Solid Edge part; units mm, degrees
sketch "Sketch1" plane through (0, 0, 0) normal (0, -1, 0) x (1, 0, 0)
  line L0 (-22.5, 45) -> (22.5, 45)
  line L1 (22.5, 45) -> (22.5, 0)
  line L2 (22.5, 0) -> (-22.5, 0)
  line L3 (-22.5, 0) -> (-22.5, 45)
  dimension "D1" = 22.5
  dimension "D2" = 22.5
  dimension "D3" = 22.5
  dimension "D4" = 22.5
extrude "Protrusion1" add sketch "Sketch1" against normal blind 270
sketch "Sketch2" plane through (22.5, 276.5897, 32.5) normal (1, 0, 0) x (0, 1, 0)
  line L0 (-86.5897, -22.5) -> (-86.5897, -32.5)
  line L1 (-86.5897, -32.5) -> (-6.5897, -32.5)
  line L2 (-6.5897, -22.5) -> (-6.5897, -32.5)
  line L3 (-86.5897, -22.5) -> (-6.5897, -22.5)
  line L4 (-276.5897, -22.5) -> (-276.5897, -32.5)
  line L5 (-196.5897, -32.5) -> (-276.5897, -32.5)
  line L6 (-196.5897, -32.5) -> (-196.5897, -22.5)
  line L7 (-196.5897, -22.5) -> (-276.5897, -22.5)
  dimension "D1" = 86.5897
  dimension "D2" = 86.5897
extrude "ExtrudedProtrusion_3" add sketch "Sketch2" along normal blind 65
sketch "Sketch3" plane through (50, 0, 15) normal (0, -1, 0) x (1, 0, 0)
  line L0 (-60, 17.5) -> (-60, 12.5)
  line L1 (-60, 12.5) -> (-55, 12.5)
  line L2 (-55, 12.5) -> (-55, 17.5)
  line L3 (-55, 17.5) -> (-60, 17.5)
extrude "ExtrudedProtrusion_5" add sketch "Sketch3" along normal blind 14.1229
sketch "Sketch4" plane through (0, -7.0615, 32.5) normal (0, 0, 1) x (0, 1, 0)
  line L0 (-7.0615, 10) -> (-7.0615, 5)
  line L1 (-7.0615, 5) -> (-2.0615, 5)
  line L2 (-2.0615, 5) -> (-2.0615, 10)
  line L3 (-2.0615, 10) -> (-7.0615, 10)
  dimension "D1" = 2.0615
extrude "ExtrudedProtrusion_6" add sketch "Sketch4" along normal blind 90
sketch "Sketch5" plane through (0, -9.1229, 61.3303) normal (0, 1, 0) x (0, 0, -1)
  line L0 (-61.1697, 10) -> (-61.1697, 5)
  line L1 (-61.1697, 5) -> (-56.1697, 5)
  line L2 (-56.1697, 5) -> (-56.1697, 10)
  line L3 (-56.1697, 10) -> (-61.1697, 10)
  dimension "D1" = 56.1697
extrude "ExtrudedProtrusion_7" add sketch "Sketch5" along normal blind 100
sketch "Sketch6" plane through (50, 270, 15) normal (0, 1, 0) x (0, 0, -1)
  line L0 (-17.5, 55) -> (-12.5, 55)
  line L1 (-12.5, 55) -> (-12.5, 60)
  line L2 (-17.5, 60) -> (-12.5, 60)
  line L3 (-17.5, 55) -> (-17.5, 60)
  dimension "D1" = 17.5
  dimension "D2" = 17.5
  dimension "D3" = 17.5
extrude "ExtrudedProtrusion_8" add sketch "Sketch6" along normal blind 14.2
sketch "Sketch7" plane through (0, 377.1, 32.5) normal (0, 0, 1) x (0, 1, 0)
  line L0 (-97.9, 10) -> (-92.9, 10)
  line L1 (-92.9, 10) -> (-92.9, 5)
  line L2 (-92.9, 5) -> (-97.9, 5)
  line L3 (-97.9, 5) -> (-97.9, 10)
  dimension "D1" = 97.9
  dimension "D2" = 92.9
extrude "ExtrudedProtrusion_9" add sketch "Sketch7" along normal blind 90
sketch "Sketch8" plane through (0, 279.2, 62.5) normal (0, -1, 0) x (0, 0, 1)
  line L0 (55, 10) -> (60, 10)
  line L1 (60, 10) -> (60, 5)
  line L2 (60, 5) -> (55, 5)
  line L3 (55, 5) -> (55, 10)
  dimension "D1" = 55
  dimension "D2" = 60
extrude "ExtrudedProtrusion_10" add sketch "Sketch8" along normal blind 100
sketch "Sketch9" plane through (-22.5, 185, 15) normal (-1, 0, 0) x (0, 1, 0)
  line L0 (-60, 15) -> (-60, -30)
  line L1 (-60, -30) -> (-40, -30)
  line L2 (-40, -30) -> (-40, 15)
  line L3 (-40, 15) -> (-60, 15)
  dimension "D1" = 60
  dimension "D2" = 40
extrude "ExtrudedProtrusion_11" add sketch "Sketch9" along normal blind 90
hole "Hole_1" at (-87.5, 125, 22.5) direction (0, 1, 0) diameter 30 end up to next
fillet "Round_1" radius 10 2 edges at (-112.5, 135, 0) (-112.5, 135, 45)
hole "Hole_2" at (-5, -11.6229, 75) direction (-1, 0, 0) diameter 3 end up to next
extrude "Protrusion2" [suppressed]
Work out the finished part from the listing and answer in its coordinate system (mm). A direction names the side the tool comes from. Round coordinates to 2 decimals unless told otherwise and drop trailing zeros. Write each loop counter-clockwise with the first axis right and the second up, starting at its lowest first coordinate (ties: lowest second). Pieces come first, ordered by that corner, then holes.
1) A cutting plane is placed at B-B on z = 22.5. Determine the outline of the cut face in (x, y), and give its area (4 significant figures).
2) Consider probe 1 along Y at (x, z) = (-7, 75); probe 2 along Z at (x, y) = (-87.5, 133.75); probe 3 along X at (y, z) = (139, 22). Determine where each line is inside the solid, lowest interval first.
3) A cutting plane is placed at C-C on x = -87.5. Determine the outline of the cut face in (y, z), and give its area (3 significant figures).
4) Which of the six approach directions +Z, -Z, +X, -X, +Y, -Y give full straight-line access (tool end or side, diameter ignored) to faces 5 (the face through (55, 190, 5)), 6 (the face through (-10, 282, 93)), 7 (the face through (55, 229, 10)), 8 (the face through (-22.5, 62, 22)), 9 (the face through (-22.5, 207, 22))?
5) Determine the mould class of faces 1 (the face through (87.5, 229, 5)), 2 (the face through (-102.143, 134.86, 25.752)), 3 (the face through (-112.5, 135, 23)), 4 (the face through (9, 0, 17)) for opening direction X: pulls with the +X half, pulls with the -X half, needs draft (parallel to the pull), parting line crosses it, or undercut.
6) Flat-ended cylindrical pins translate along their axes: P1, Ø4, axis at y = 95.5, z = 17, coming from the -X side; P2, Ø10, axis at y = 227.5, z = 41.5, coming from the +X side; P3, Ø13.5, axis at x = 41.5, z = 17.5, coming from the +Y side; P4, Ø1.5, axis at x = -6.5, y = -10, coming from the -Z side. Find the tip coordinate at first contact, or state that the pin passes through.
7) A cutting plane is placed at A-A on y = 223.5. Determine the outline of the cut face in (x, z).
8) A cutting plane is placed at D-D on y = 141.5. Determine the outline of the cut face in (x, z), and give its area (3 significant figures).
Entries:
1. outline: (-112.5, 125) - (-102.5, 125) - (-102.5, 145) - (-112.5, 145) - close; (-72.5, 125) - (-22.5, 125) - (-22.5, 0) - (22.5, 0) - (22.5, 270) - (-22.5, 270) - (-22.5, 145) - (-72.5, 145) - close
1. area: 13,350 mm2
2. probe 1: y = -14.12 to -13.12, -10.12 to -9.12, 279.2 to 284.2
2. probe 2: z = 0 to 7.5, 37.5 to 45
2. probe 3: x = -112.5 to -102.49, -72.51 to 22.5
3. outline: (125, 0) - (145, 0) - (145, 7.5) - (125, 7.5) - close; (125, 37.5) - (145, 37.5) - (145, 45) - (125, 45) - close
3. area: 300 mm2
4. face 5: +Z, -Z, +X
4. face 6: +Z, -X, +Y
4. face 7: +Z, +X, +Y, -Y
4. face 8: +Z, -Z, -X, -Y
4. face 9: +Z, -Z, -X, +Y
5. face 1: pulls with the +X half
5. face 2: undercut
5. face 3: pulls with the -X half
5. face 4: needs draft
6. P1: stops at x = -22.5
6. P2: stops at x = 22.5
6. P3: passes through
6. P4: stops at z = 27.5
7. outline: (-22.5, 0) - (87.5, 0) - (87.5, 10) - (22.5, 10) - (22.5, 45) - (-22.5, 45) - close; (-10, 117.5) - (-5, 117.5) - (-5, 122.5) - (-10, 122.5) - close
8. outline: (-112.5, 10) arc R10 ccw to (-102.5, 0) - (22.5, 0) - (22.5, 45) - (-102.5, 45) arc R10 ccw to (-112.5, 35) - close; hole circle Ø30 at (-87.5, 22.5)
8. area: 5,330 mm2
